Part print with two shaded views. Sizes in mm from the minimum x, y, z corner. Give positions to 0.01 mm unless a question says otherwise; leave off trailing zeros. Loops run counter-clockwise (first coordinate to the right, second up) from the corner with the lowest first, then second, coordinate; pieces in that order, holes last. Notation, with made-up numbers: (-37.75, -38.5) -> (-11.75, -38.5) arc R23 cw to (-11.75, -16.5) -> close; hole circle Ø5 at (12, 54). An arc over 180 degrees is marked (long way). One line per question, with ' | ' between items.
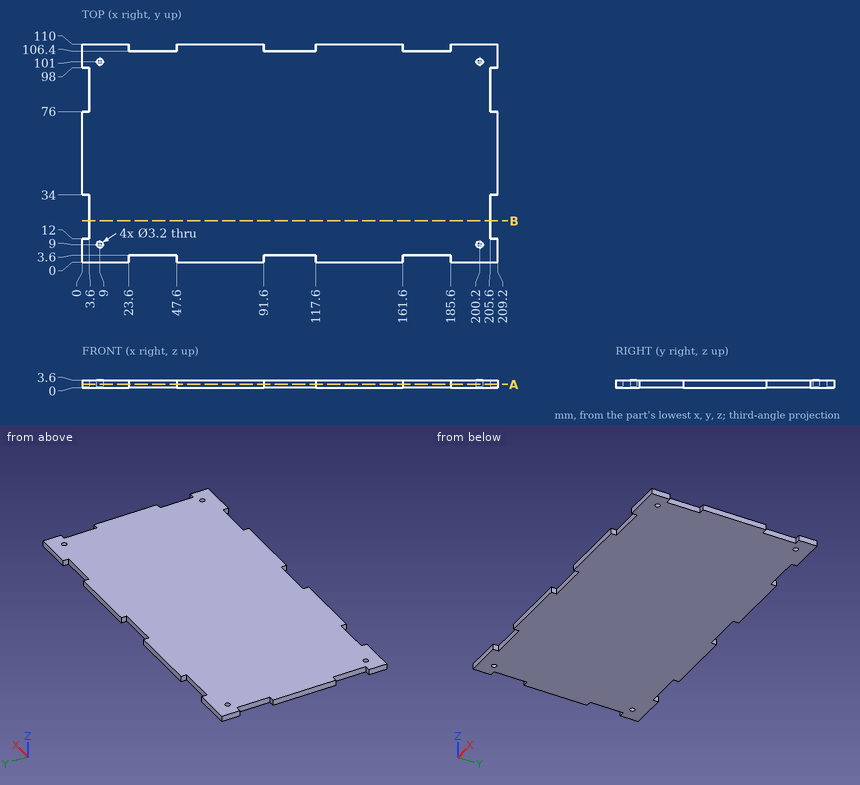
1) Drill centre lines: line 1 (Y direction, x = 9, z = 1.6); line 2 (X direction, y = 101, z = 2.3); line 3 (X direction, y = 93, z = 1.35). Where is each one in solid material? Low to high.
Found:
line 1: 0 to 7.4, 10.6 to 99.4, 102.6 to 110 | line 2: 0 to 7.4, 10.6 to 198.6, 201.8 to 209.2 | line 3: 3.6 to 205.6
2) Saw through at B-B (y = 21). Give the cut face in (x, z), and give its area (3 significant figures).
Found:
outline: (3.6, 0) -> (205.6, 0) -> (205.6, 3.6) -> (3.6, 3.6) -> close | area: 727 mm2
3) Pin check, flat tips, straight feed: P1, Ø1.1, axis at x = 175, z = 1.5, coming from the -Y side; P2, Ø1.1, axis at x = 106.5, z = 2.5, coming from the +Y side; P3, Ø2, axis at y = 32.5, z = 1, coming from the -X side. Stop position of each tip, or through.
Found:
P1: y = 3.6 | P2: y = 106.4 | P3: x = 3.6
4) Saw through at A-A (z = 1.6). State how many separate pieces and enclosed holes the cut face has, and give its area (3 significant figures).
Found:
separate pieces: 1 | enclosed holes: 4 | area: 22,100 mm2
